Autodesk Inventor part; units mm, degrees
ref_plane "YZ Plane" through (0, 0, 0) normal (1, 0, 0) x (0, 1, 0)
ref_plane "XZ Plane" through (0, 0, 0) normal (0, 1, 0) x (-1, 0, 0)
ref_plane "XY Plane" through (0, 0, 0) normal (0, 0, 1) x (1, 0, 0)
sketch "Sketch1" plane through (0, 0, 0) normal (0, 0, 1) x (1, 0, 0)
  circle A0 centre (0, 0) radius 48
  circle A1 centre (141.8, 0) radius 60.5
  line L0 (136.466784, 60.264474) -> (-4.231312, 47.813136)
  line L1 (-4.231312, -47.813136) -> (136.466784, -60.264474)
  line L2 (80.8, 55.338139) -> (80.8, -55.338139)
  dimension "d0" = 96
  dimension "d1" = 121
  dimension "d2" = 141.8
  dimension "d3" = 61
extrude "Extrusion1" add sketch "Sketch1" against normal blind 21 contours L0 A1 L1 L2 | A1
sketch "Sketch2" plane through (0, 0, -21) normal (0, 0, -1) x (-1, 0, 0)
  line L0 (-80.8, -55.338139) -> (-60.3, -53.523954)
  line L1 (-60.3, -53.523954) -> (-60.3, 53.523954)
  line L2 (-60.3, 53.523954) -> (-80.8, 55.338139)
  line L3 (-80.8, 55.338139) -> (-80.8, -55.338139)
  line L4 (-136.466784, -60.264474) -> (-80.8, -55.338139)
  line L5 (-80.8, 55.338139) -> (-136.466784, 60.264474)
  line L6 (-80.8, -55.338139) -> (-80.8, 55.338139)
  point P0 (0, 0)
  dimension "d7" = 20.5
extrude "Extrusion2" add sketch "Sketch2" against normal blind 12
shell "Shell1" thickness 4 removed faces 1 at (111.077856, 17.841318, -21)
sketch "Sketch3" plane through (141.8, 0, -4) normal (0, 0, -1) x (-1, 0, 0)
  circle A0 centre (0, 0) radius 42
  point P0 (141.8, 0)
  dimension "d10" = 84
extrude "Extrusion3" cut sketch "Sketch3" against normal blind 1
sketch "Sketch4" plane through (0, 0, 0) normal (0, 0, 1) x (1, 0, 0)
  circle A0 centre (141.8, 0) radius 42
  circle A1 centre (141.8, 0) radius 35.5
  point P0 (0, 0)
  dimension "d13" = 71
extrude "Extrusion4" cut sketch "Sketch4" against normal through all contours A1
sketch "Sketch5" plane through (141.8, 0, -4) normal (0, 0, -1) x (-1, 0, 0)
  circle A0 centre (0, 0) radius 45
  circle A1 centre (0, 0) radius 48
  point P0 (141.8, 0)
  dimension "d16" = 90
  dimension "d17" = 96
extrude "Extrusion5" add sketch "Sketch5" along normal blind 9
sketch "Sketch6" plane through (84.8, -51.676494, -13) normal (0, 0, -1) x (-1, 0, 0)
  line L0 (8.632076, 0.763912) -> (62.461619, 5.527656)
  line L1 (62.461619, 5.527656) -> (62.461619, 97.825331)
  line L2 (62.461619, 97.825331) -> (8.632076, 102.589076)
  line L3 (8.632076, 102.589076) -> (8.632076, 0.763912)
  line L4 (20.5, 1.814185) -> (-52.019394, -4.603552)
  line L5 (-52.019394, 107.956539) -> (20.5, 101.538802)
extrude "Extrusion6" cut sketch "Sketch6" along normal through all
fillet "Fillet1" radius 4 3 edges at (84.8, 0, -13) (80.8, 0, -9) (80.8, 0, 0)
sketch "Sketch7" plane through (141.8, 0, -4) normal (0, 0, -1) x (-1, 0, 0)
  line L0 (-52, 4) -> (-60, 4)
  line L1 (-60, 4) -> (-60, -4)
  line L2 (-60, -4) -> (-52, -4)
  line L3 (-52, -4) -> (-52, 4)
  line L4 (-52, 4) -> (-60, -4) construction
  line L5 (-60, 4) -> (-52, -4) construction
  arc A0 (4.980606, 56.280046) -> (4.980606, -56.280046) centre (0, 0) ccw
  line L6 (4.980606, -56.280046) -> (12.949463, -55.574827)
  line L7 (12.949463, -55.574827) -> (12.596853, -51.590399)
  line L8 (12.596853, -51.590399) -> (4.627997, -52.295618)
  line L9 (4.627997, -52.295618) -> (4.980606, -56.280046)
  line L10 (4.980606, 56.280046) -> (57, 51.676494)
  line L11 (4.980606, 56.280046) -> (12.949463, 55.574827)
  line L12 (12.949463, 55.574827) -> (12.596853, 51.590399)
  line L13 (12.596853, 51.590399) -> (4.627997, 52.295618)
  line L14 (4.627997, 52.295618) -> (4.980606, 56.280046)
  point P0 (141.8, 0)
  point P1 (-56, 0)
  dimension "d24" = 4
  dimension "d25" = 4
  dimension "d26" = 8
  dimension "d27" = 8
  dimension "d28" = 8
  dimension "d29" = 56
extrude "Extrusion7" add sketch "Sketch7" along normal up to surface (17 mm away)
sketch "Sketch8" plane through (0, 0, 0) normal (0, 0, -1) x (-1, 0, 0)
  line L0 (-60.3, -49.508321) -> (-128.850537, -55.574827)
  line L1 (-128.850537, 55.574827) -> (-60.3, 49.508321)
  circle A0 centre (-141.8, 0) radius 35.5
  line L2 (-128.850537, -55.574827) -> (-129.203147, -51.590399)
  line L3 (-129.203147, 51.590399) -> (-128.850537, 55.574827)
  point P0 (0, 0)
  point P1 (-197.8, 0)
  point P2 (-132.834965, -55.927437)
  point P3 (-132.834965, 55.927437)
  dimension "d32" = 56
  dimension "d33" = 4
  dimension "d34" = 4
hole "Hole1" at (197.8, 0, 0) at (132.834965, -55.927437, 0) at (132.834965, 55.927437, 0) direction (0, 0, -1) diameter 3.4 end through all counterbore diameter 6.5 counterbore depth 17
sketch "Sketch9" plane through (0, 0, 0) normal (0, 0, 1) x (1, 0, 0)
  circle A0 centre (125.937089, 54.374793) radius 1.7
  circle A1 centre (132.834965, -55.927437) radius 1.7
  circle A2 centre (197.8, 0) radius 1.7
  point P0 (0, 0)
equation "\"d25\" = d24"
equation "\"d27\" = d26"
equation "\"d28\" = d26"
properties part number "J1-sketch"
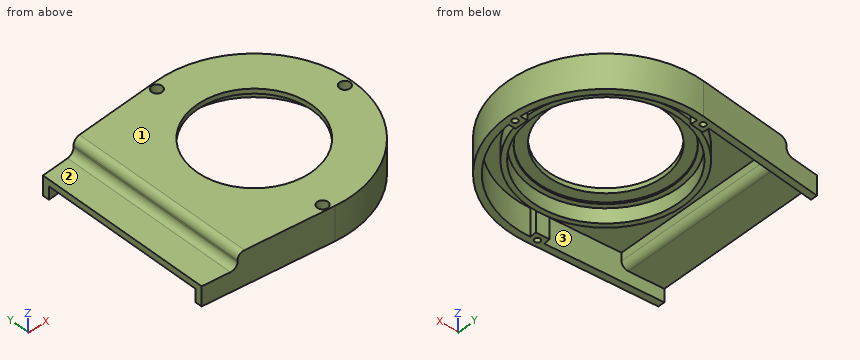
Check sheet for the modelled part. Datum: model origin and axes. Units: mm. Face numbers are marked on the shaded views. A direction names the side the tool comes from. Coordinates: 2 decimals unless noted, no trailing zeros. Write each loop counter-clockwise with the first axis right and the second up, starting at its lowest first coordinate (ties: lowest second). Pieces come first, ordered by that corner, then holes. Notation, with made-up numbers: (79, 73) - (106, 73) arc R31 ccw to (106, 107) - close; hole circle Ø11 at (59.25, -37). An arc over 180 degrees is marked (long way). One line per question, with ' | ' between items.
Item 1: Access from +Z, -Z, +X, -X, +Y, -Y to the whole of each face (thin tool, end or side, straight path). Record for the marked faces 1, 2 and 3.
Determined:
face 1: +Z, +X, -X, +Y, -Y | face 2: +Z, -X, +Y, -Y | face 3: -Z
Item 2: Sectioned sample at B-B on z = -7. Record the boundary of the cut face in (x, y), plus the area to 3 significant figures.
Determined:
outline: (80.26, -55.29) - (136.47, -60.26) arc R60.5 ccw (long way) to (136.47, 60.26) - (80.26, 55.29) - close; circle Ø96 at (141.8, 0); hole (84.8, -51.68) - (128.85, -55.57) - (129.2, -51.59) - (137.17, -52.3) - (136.82, -56.28) arc R56.5 ccw to (198.16, -4) - (193.8, -4) - (193.8, 4) - (198.16, 4) arc R56.5 ccw to (136.82, 56.28) - (137.17, 52.3) - (129.2, 51.59) - (128.85, 55.57) - (84.8, 51.68) - close; hole circle Ø90 at (141.8, 0); hole circle Ø6.5 at (132.83, -55.93); hole circle Ø6.5 at (132.83, 55.93); hole circle Ø6.5 at (197.8, 0) | area: 2,570 mm2
Item 3: Sectioned sample at A-A on x = 141.8. Record the boundary of the cut face in (y, z).
Determined:
outline: (-60.5, -21) - (-56.5, -21) - (-56.5, -4) - (-48, -4) - (-48, -13) - (-45, -13) - (-45, -4) - (-42, -4) - (-42, -3) - (-35.5, -3) - (-35.5, 0) - (-60.5, 0) - close; (35.5, -3) - (42, -3) - (42, -4) - (45, -4) - (45, -13) - (48, -13) - (48, -4) - (56.5, -4) - (56.5, -21) - (60.5, -21) - (60.5, 0) - (35.5, 0) - close
Item 4: Thickness scan on line 1 (Y direction, x = 141.8, z = -10); line 2 (X direction, y = -34, z = -12); line 3 (X direction, y = 7.5, z = -9.5). Record the ranges inside material, lowest first. Write a range as [from, to].
Determined:
line 1: y = [-60.5, -56.5], [-48, -45], [45, 48], [56.5, 60.5] | line 2: x = [60.3, 83.45], [107.92, 112.32], [171.28, 175.68], [186.92, 191.84] | line 3: x = [60.3, 84.77], [94.39, 97.43], [186.17, 189.21], [197.8, 201.83]
Item 5: Sectioned sample at D-D on z = -15.25. Record the boundary of the cut face in (x, y), plus the area to 3 significant figures.
Determined:
outline: (60.3, -53.52) - (136.47, -60.26) arc R60.5 ccw (long way) to (136.47, 60.26) - (60.3, 53.52) - (60.3, 49.51) - (128.85, 55.57) - (129.2, 51.59) - (137.17, 52.3) - (136.82, 56.28) arc R56.5 cw to (198.16, 4) - (193.8, 4) - (193.8, -4) - (198.16, -4) arc R56.5 cw to (136.82, -56.28) - (137.17, -52.3) - (129.2, -51.59) - (128.85, -55.57) - (60.3, -49.51) - close; hole circle Ø6.5 at (132.83, -55.93); hole circle Ø6.5 at (132.83, 55.93); hole circle Ø6.5 at (197.8, 0) | area: 1,390 mm2
Item 6: Gauge pin test, flat ends, axial feed: P1, Ø4, axis at x = 132.83, y = 55.93, coming from the +Z side; P2, Ø2, axis at x = 169, z = -6.5, coming from the +Y side; P3, Ø1.5, axis at y = -21.5, z = -7, coming from the +X side. Record the tip position at first contact, or that the pin passes through.
Determined:
P1: stops at z = -17 | P2: stops at y = 54.53 | P3: stops at x = 198.63
